Check sheet for the modelled part. Datum: model origin and axes. Units: mm. Face numbers are marked on the shaded views. A direction names the side the tool comes from. Round coordinates to 2 decimals unless told otherwise and drop trailing zeros. Loops run counter-clockwise (first coordinate to the right, second up) from the corner with the lowest first, then second, coordinate; pieces in that order, holes last. Notation, with made-up numbers: M 57,22.5 L 72,22.5 A34 ccw 72,61.5 Z; hole C -18.75,-11.75 d5. An arc over 180 degrees is marked long. One line per question, with ' | ' between items. Start each with the question number.
(1) Section check B-B (z = -73.5). Record the boundary of the cut face in (x, y), and give its area (3 significant figures).
(2) Section check C-C (y = -116.5). Record the boundary of the cut face in (x, z), and give its area (3 significant figures).
(3) Thickness scan on probe 1 along Z at (x, y) = (-6, -448); probe 2 along X at (y, z) = (-26, -123.5); probe 3 along Z at (x, y) = (-0.75, -94.5). Record the ranges inside material, lowest first. Write a range as [from, to].
(4) Section check A-A (x = -2). Record the boundary of the cut face in (y, z).
(5) Tool access check on the marked faces 1 and 2. Record the directions out of +Z, -Z, +X, -X, +Y, -Y that give a thin tool (end or side, any length) a straight path to the whole face; none if there is none.
(6) Go/stop test with flat-tipped pins: P1, Ø3, axis at x = -0.5, y = -248.5, coming from the -Z side; P2, Ø3.5, axis at x = 2, y = -249.5, coming from the -Z side; P3, Ø1, axis at x = -5.5, z = -68, coming from the -Y side; P4, Ø3.5, axis at x = -5, y = -225, coming from the -Z side. Record where each tip stops, or that it passes through.
(7) Section check D-D (y = -429). Record the boundary of the cut face in (x, z).
```python
from build123d import *

# Parameters (mm, degrees)
F1_DEPTH = 505
F2_W     = 10
F2_H     = 10
F3_DEPTH = 2
F5_DEPTH = 25
F7_DEPTH = 25
F8_R     = 5


with BuildPart() as f1:
    # F0 (on Front) → F1 (new body)
    with BuildSketch(Plane.XZ):
        Polygon((3, 5.9644671453), (-7, 5.9644671453), (-7, 2.8680202551), (-4, 2.8680202551), (-4, -147.1319797449), (0, -147.1319797449), (0, 2.8680202551), (3, 2.8680202551), align=None)
    extrude(amount=F1_DEPTH)

    # F2 (on face) → F3 (join)
    with BuildSketch(Plane.XY.offset(5.9644671453)):
        with Locations((-2, -500)):
            Rectangle(F2_W, F2_H)
    extrude(amount=F3_DEPTH)

    # F4 (on face) → F5 (cut)
    with BuildSketch(Plane(origin=(-4, 0, 0), x_dir=(0, -1, 0), z_dir=(-1, 0, 0))):
        Polygon((505, -147.1319797449), (505, -7.1319797449), (0, -147.1319797449), align=None)
    extrude(amount=-F5_DEPTH, mode=Mode.SUBTRACT)

    # F6 (on face) → F7 (cut)
    with BuildSketch(Plane(origin=(-4, 0, 0), x_dir=(0, -1, 0), z_dir=(-1, 0, 0))):
        Polygon((452.3232281555, -5.1319797449), (2, -5.1319797449), (2, -129.9740627979), align=None)
    extrude(amount=-F7_DEPTH, mode=Mode.SUBTRACT)

    # F8
    f8_edges = [f1.edges().sort_by_distance(p)[0] for p in [
        (-2, -2, -5.13198),
        (-2, -452.323228, -5.13198),
    ]]
    fillet(f8_edges, radius=F8_R)


solid = f1.part
```
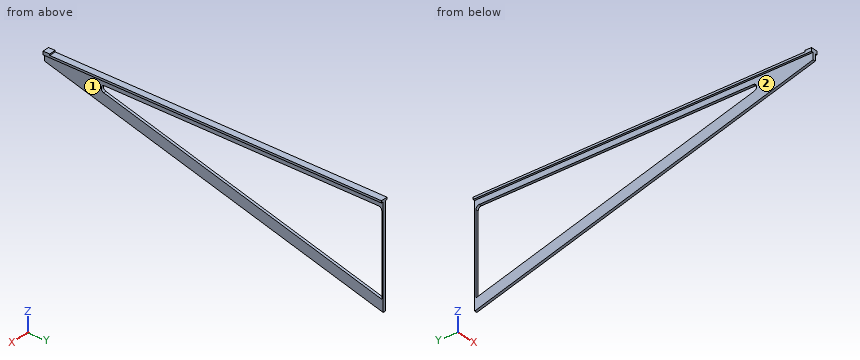
The answers:
1) outline: M -4,-265.6 L 0,-265.6 L 0,-205.71 L -4,-205.71 Z; M -4,-2 L 0,-2 L 0,0 L -4,0 Z | area: 248 mm²
2) outline: M -7,2.87 L -4,2.87 L -4,-5.13 L 0,-5.13 L 0,2.87 L 3,2.87 L 3,5.96 L -7,5.96 Z; M -4,-114.83 L 0,-114.83 L 0,-98.23 L -4,-98.23 Z | area: 129 mm²
3) probe 1: [2.87, 5.96] | probe 2: [-4, 0] | probe 3: [-120.93, -104.33], [-5.13, 5.96]
4) outline: M -505,-7.13 L 0,-147.13 L 0,5.96 L -495,5.96 L -495,7.96 L -505,7.96 Z; hole M -416.91,-14.95 L -2,-129.97 L -2,-10.13 A5 ccw -7,-5.13 L -415.57,-5.13 A5 ccw Z
5) face 1: -Z, +X, +Y, -Y | face 2: -Z, -X, +Y, -Y
6) P1: z = -78.66 | P2: z = 2.87 | P3: through | P4: z = -85.15
7) outline: M -7,2.87 L -4,2.87 L -4,-28.2 L 0,-28.2 L 0,2.87 L 3,2.87 L 3,5.96 L -7,5.96 Z
